CAD build for the part. Positions are in the model's coordinates, mm. A direction names the side the tool comes from. Give positions to 0.01 mm unless a question says otherwise; leave off trailing zeros. Write each loop counter-clockwise with the first axis right and the second up, starting at its lowest first coordinate (ties: lowest second). Pieces come first, ordered by that corner, then holes. Notation, with made-up numbers: M 56.5,20.25 L 93.5,20.25 A35 ccw 93.5,58.25 Z; hole C 62.5,-14 d4. An arc over 180 degrees is marked long. One line per question, with ' | ' between items. Start each with the question number.
1. Cut at A-A, the plane z = 107.5. Write the cut outline in (x, y).
2. Cut at D-D, the plane x = -61. Write the cut outline in (y, z).
3. Pull direction Z, two halves, no side cores. Call faces 6 (the face through (35.524, 108.217, 552.414)), 7 (the face through (-2, 63, 609.6)), 8 (the face through (55, 127, 215)), 9 (the face through (-2, 27, -190.5)): released by +Z, released by -Z, zero draft, split by the parting line, or undercut.
4. Which spindle directions (+Z, -Z, +X, -X, +Y, -Y) get a long thin tool onto all of the face, cutting with end or side? Do faces 1 (the face through (-92.81, -33.9, -209.28)), 2 (the face through (101, 101, -228.6)), 3 (the face through (-1, 57, 581.9)), 4 (the face through (50.8, 108, 291)), 5 (the face through (-104, 0, 161)). Say none if no direction does.
5. Wall check: L1, parallel to X at y = 103, z = 136.5; L2, parallel to X at y = 69.5, z = 196.5; L3, parallel to Z at x = 40, y = 15. Give the ranges that are in metal, low to high.
6. Flat gauge pins, fed straight in: pin 1 (20.5 mm diameter, centred on x = 4, y = 13.5, fed in from -Z); pin 2 (6 mm diameter, centred on x = 99, z = -117, fed in from -Y). Where does each tip first touch, or does it go through?
7. Cut at B-B, the plane x = 14. Write the cut outline in (y, z), then the cut area to 3 significant figures.
8. Cut at C-C, the plane y = 49.5. Write the cut outline in (x, z).
```python
from build123d import *

# Parameters (mm, degrees)
F0_W     = 254
F0_H     = 736.6
F0_W_2   = 203.2
F0_H_2   = 596.9
F0_W_3   = 139.7
F0_H_3   = 571.5
F0_W_4   = 101.6
F0_H_4   = 546.1
F0_H_5   = 63.5
F1_DEPTH = 127
F2_DEPTH = 25.4
F3_DEPTH = 88.9
F4_R     = 50.79999
F5_DEPTH = 76.2
F6_R     = 19.05
F7_DEPTH = 38.1


# Not quite as in the source:
# - a fillet or chamfer is up to 0.001 mm smaller than in the source, because OpenCascade refuses the exact size
# - a feature names something its author has since deleted; it is built from what else it names


with BuildPart() as f1:
    # F0 (on Front) → F1 (new body)
    with BuildSketch(Plane.XZ):
        with Locations((0, 241.3)):
            Rectangle(F0_W, F0_H)
        with Locations((0, 298.45)):
            Rectangle(F0_W_2, F0_H_2, mode=Mode.SUBTRACT)
        with Locations((0, 298.45)):
            Rectangle(F0_W_2, F0_H_2)
        with Locations((0, 296.15)):
            Rectangle(F0_W_3, F0_H_3, mode=Mode.SUBTRACT)
        with Locations((0, 296.15)):
            Rectangle(F0_W_3, F0_H_3)
        with Locations((0, 293.85)):
            Rectangle(F0_W_4, F0_H_4, mode=Mode.SUBTRACT)
        with Locations((0, -158.75)):
            Rectangle(F0_W, F0_H_5)
    extrude(amount=-F1_DEPTH)

    # F0 (on Front) → F2 (cut)
    with BuildSketch(Plane.XZ):
        with Locations((0, 298.45)):
            Rectangle(F0_W_2, F0_H_2)
        with Locations((0, 296.15)):
            Rectangle(F0_W_3, F0_H_3, mode=Mode.SUBTRACT)
    extrude(amount=-F2_DEPTH, mode=Mode.SUBTRACT)

    # F0 (on Front) → F3 (cut)
    with BuildSketch(Plane.XZ):
        with Locations((0, 296.15)):
            Rectangle(F0_W_3, F0_H_3)
        with Locations((0, 293.85)):
            Rectangle(F0_W_4, F0_H_4, mode=Mode.SUBTRACT)
    extrude(amount=-F3_DEPTH, mode=Mode.SUBTRACT)

    # F4 (radius 50.8 in the source; OpenCascade refuses exactly that, so slightly less here)
    f4_edges = [f1.edges().sort_by_distance(p)[0] for p in [
        (50.8, 107.95, 566.9),
        (-50.8, 107.95, 566.9),
        (-50.8, 107.95, 20.8),
        (50.8, 107.95, 20.8),
    ]]
    fillet(f4_edges, radius=F4_R)

    # F0 (on Front) → F5 (join)
    with BuildSketch(Plane.XZ):
        with Locations((0, -158.75)):
            Rectangle(F0_W, F0_H_5)
    extrude(amount=F5_DEPTH)

    # F6 (on face) → F7 (join)
    with BuildSketch(Plane(origin=(0, 0, -190.5), x_dir=(1, 0, 0), z_dir=(0, 0, -1))):
        with Locations((-101.6, 50.8)):
            Circle(F6_R)
        with Locations((101.6, 50.8)):
            Circle(F6_R)
        with Locations((-101.6, -101.6)):
            Circle(F6_R)
        with Locations((101.6, -101.6)):
            Circle(F6_R)
    extrude(amount=F7_DEPTH)


solid = f1.part
```
Here are the results:
1) outline: M -127,0 L -101.6,0 L -101.6,25.4 L -69.85,25.4 L -69.85,88.9 L -50.8,88.9 L -50.8,127 L -127,127 Z; M 50.8,88.9 L 69.85,88.9 L 69.85,25.4 L 101.6,25.4 L 101.6,0 L 127,0 L 127,127 L 50.8,127 Z
2) outline: M -76.2,-190.5 L 127,-190.5 L 127,609.6 L 0,609.6 L 0,596.9 L 25.4,596.9 L 25.4,581.9 L 88.9,581.9 L 88.9,10.4 L 25.4,10.4 L 25.4,0 L 0,0 L 0,-127 L -76.2,-127 Z
3) face 6: undercut | face 7: released by +Z | face 8: zero draft | face 9: released by -Z
4) face 1: -Z | face 2: -Z, +X, -X, +Y, -Y | face 3: -Y | face 4: +Y, -Y | face 5: +Z, +X, -X, -Y
5) L1: -127 to -50.8, 50.8 to 127 | L2: -127 to -69.85, 69.85 to 127 | L3: -190.5 to 0, 596.9 to 609.6
6) pin 1: z = -190.5 | pin 2: y = 0
7) outline: M -76.2,-190.5 L 127,-190.5 L 127,22.77 L 88.9,22.77 L 88.9,10.4 L 25.4,10.4 L 25.4,0 L 0,0 L 0,-127 L -76.2,-127 Z; M 0,596.9 L 25.4,596.9 L 25.4,581.9 L 88.9,581.9 L 88.9,564.93 L 127,564.93 L 127,609.6 L 0,609.6 Z | area: 34,300 mm^2
8) outline: M -127,-190.5 L 127,-190.5 L 127,609.6 L -127,609.6 Z; hole M -69.85,10.4 L 69.85,10.4 L 69.85,581.9 L -69.85,581.9 Z
